Geometry check sheet. Reference: the model listing, model coordinates, mm. A direction names the side the tool comes from. Coordinates: 2 decimals unless noted, no trailing zeros. Loops run counter-clockwise (first coordinate to the right, second up) from the corner with the lowest first, then second, coordinate; pieces in that order, holes last. Notation, with made-up numbers: M 76.5,2 L 125.5,2 A23 ccw 125.5,18 Z; hole C 80.5,38 d4. An arc over 180 degrees is marked long. One line per question, with ' | ' between items. Start each with the question number.
from build123d import *

# Parameters (mm, degrees)
EXTRUDE_354_DEPTH      = 3
CUT_EXTRUDE_1082_REACH = 143.453
SKETCH_3_W             = 15
SKETCH_3_H             = 10
SKETCH_4_R             = 3
SKETCH_4_R_2           = 1.5
EXTRUDE_1381_DEPTH     = 8
SKETCH_5_W             = 83
SKETCH_5_H             = 5
EXTRUDE_1698_DEPTH     = 45
SKETCH_6_W             = 2
SKETCH_6_H             = 5
CUT_EXTRUDE_1867_DEPTH = 83
SKETCH_7_W             = 40
SKETCH_7_H             = 13
TYPE_C_DEPTH           = 3
SKETCH_8_W             = 10
SKETCH_8_H             = 5
CUT_EXTRUDE_3_DEPTH    = 2
SKETCH_9_W             = 11
SKETCH_9_H             = 20
CUT_EXTRUDE_4_DEPTH    = 3
EXTRUDE_START          = -83
EXTRUDE_1_DEPTH        = 83
SKETCH_2_3_R           = 1.5
CUT_EXTRUDE_5_DEPTH    = 10


with BuildPart() as part:
    # 草图1 → Extrude 354 (new body)
    with BuildSketch(Plane(origin=(0, 0, 0), x_dir=(1, 0, 0), z_dir=(0, 1, 0))):
        with BuildLine():
            Line((3, 0), (97, 0))
            ThreePointArc((97, 0), (99.121320344, 0.878679656), (100, 3))
            Line((100, 3), (100, 97))
            ThreePointArc((100, 97), (99.121320344, 99.121320344), (97, 100))
            Line((97, 100), (3, 100))
            ThreePointArc((3, 100), (0.878679656, 99.121320344), (0, 97))
            Line((0, 97), (0, 3))
            ThreePointArc((0, 3), (0.878679656, 0.878679656), (3, 0))
        make_face()
    extrude(amount=EXTRUDE_354_DEPTH)

    # 草图3 → Cut-Extrude 1082 (cut, up to next)
    with BuildSketch(Plane(origin=(0, 3, 0), x_dir=(1, 0, 0), z_dir=(0, 1, 0)), mode=Mode.PRIVATE) as cut_extrude_1082_sk1:
        with Locations((50, 50)):
            Rectangle(SKETCH_3_W, SKETCH_3_H)
    cut_extrude_1082_tool1 = extrude(cut_extrude_1082_sk1.sketch, amount=-CUT_EXTRUDE_1082_REACH, mode=Mode.PRIVATE) & part.part
    add(cut_extrude_1082_tool1.solids().sort_by_distance((50, 3, -50))[0], mode=Mode.SUBTRACT)

    # 草图4 → Extrude 1381 (add)
    with BuildSketch(Plane.XZ):
        with Locations(Location((50, -30, 0), (0, 0, 270))):
            Circle(SKETCH_4_R)
        with Locations(Location((50, -30, 0), (0, 0, 270))):
            Circle(SKETCH_4_R_2, mode=Mode.SUBTRACT)
    extrude(amount=EXTRUDE_1381_DEPTH)

    # 草图5 → Extrude 1698 (add)
    with BuildSketch(Plane.XZ):
        with Locations((50, -97.5)):
            Rectangle(SKETCH_5_W, SKETCH_5_H)
    extrude(amount=EXTRUDE_1698_DEPTH)

    # 草图6 → Cut-Extrude 1867 (cut)
    with BuildSketch(Plane(origin=(91.5, 0, 0), x_dir=(0, 0, -1), z_dir=(1, 0, 0))):
        with Locations((99, -42.5)):
            Rectangle(SKETCH_6_W, SKETCH_6_H)
    extrude(amount=-CUT_EXTRUDE_1867_DEPTH, mode=Mode.SUBTRACT)

    # 草图7 → TYPE-C板口 (cut)
    with BuildSketch(Plane.XY.offset(-95)):
        with Locations((50, -38.5)):
            Rectangle(SKETCH_7_W, SKETCH_7_H)
    extrude(amount=-TYPE_C_DEPTH, mode=Mode.SUBTRACT)

    # 草图8 → 切除-拉伸3 (cut)
    with BuildSketch(Plane.XY.offset(-98)):
        with Locations((50, -37.5)):
            Rectangle(SKETCH_8_W, SKETCH_8_H)
    extrude(amount=-CUT_EXTRUDE_3_DEPTH, mode=Mode.SUBTRACT)

    # 草图9 → 切除-拉伸4 (cut)
    with BuildSketch(Plane.XY.offset(-95)):
        with Locations((86, -17.5)):
            Rectangle(SKETCH_9_W, SKETCH_9_H)
        with Locations((14, -17.5)):
            Rectangle(SKETCH_9_W, SKETCH_9_H)
    extrude(amount=-CUT_EXTRUDE_4_DEPTH, mode=Mode.SUBTRACT)

    # 草图10 → 凸台-拉伸1 (add)
    with BuildSketch(Plane(origin=(91.5, 0, 0), x_dir=(0, 0, -1), z_dir=(1, 0, 0)).offset(EXTRUDE_START)):
        Polygon((95, -7.5), (98, -9.5), (98, -7.5), align=None)
        Polygon((95, -27.5), (98, -25.5), (98, -27.5), align=None)
    extrude(amount=EXTRUDE_1_DEPTH)

    # 放样2: read off the stored shape, not the designer's step
    # 放样2: loft between two sections, ruled curve by curve
    loft_2_from = [
        Edge.make_bspline([(19.446610657, 0, -55.974425515), (31.395461687, 0, -57.081204201), (32.502240373, 0, -45.132353171), (20.553389343, 0, -44.025574485), (8.604538313, 0, -42.918795799), (7.497759627, 0, -54.867646829), (19.446610657, 0, -55.974425515)], [0, 0, 0, 0, 0.5, 0.5, 0.5, 1, 1, 1, 1], 3, [1, 0.333333333, 0.333333333, 1, 0.333333333, 0.333333333, 1]),
    ]
    loft_2_to = [
        Edge.make_bspline([(18.541542898, -10, -52.621622185), (23.784787268, -10, -55.538536389), (26.701701472, -10, -50.295292019), (21.458457102, -10, -47.378377815), (16.215212732, -10, -44.461463611), (13.298298528, -10, -49.704707981), (18.541542898, -10, -52.621622185)], [0, 0, 0, 0, 0.5, 0.5, 0.5, 1, 1, 1, 1], 3, [1, 0.333333333, 0.333333333, 1, 0.333333333, 0.333333333, 1]),
    ]
    loft_2 = Solid(Shell([*[Face.make_surface_from_curves(loft_2_from[k], loft_2_to[k]) for k in range(1)], Face(Wire(loft_2_from)), Face(Wire(loft_2_to))]))
    add(loft_2)

    # 草图2<3> → 切除-拉伸5 (cut)
    with BuildSketch(Plane.XZ.offset(10)):
        with Locations(Location((20, -50, 0), (0, 0, 270))):
            Circle(SKETCH_2_3_R)
    cut_extrude_5 = extrude(amount=-CUT_EXTRUDE_5_DEPTH, mode=Mode.SUBTRACT)

    # 镜向1: 放样2, 切除-拉伸5 across plane
    add(loft_2.mirror(Plane.ZY.offset(-50)))
    add(cut_extrude_5.mirror(Plane.ZY.offset(-50)), mode=Mode.SUBTRACT)


solid = part.part
1. Thickness scan on line 1 (Z direction, x = 80, y = -1.75); line 2 (X direction, y = -7.5, z = -50); line 3 (X direction, y = -6, z = -50). Record the ranges inside material, lowest first.
2. Tool access check on faces 4 (the flat face through (13.9, -26.5, -96.5)), 5 (the flat face through (50, -32, -96)), 6 (the flat face through (91.5, -22, -99)). Record the directions out of +Z, -Z, +X, -X, +Y, -Y that give a thin tool (end or side, any length) a straight path to the whole face; none if there is none.
3. Sectioned sample at C-C (z = -30). Record the cut outline in (x, y).
4. Draft check along Y on faces 1 (the flat face through (19, -45, -96)), 2 (the flat face through (85.9, -26.5, -96.5)), 3 (the flat face through (51, -19, -100)). Enter one of: +Y half, -Y half, draft (parallel to the pull), parting line (faces both ways), or undercut.
5. Sectioned sample at A-A (x = 50). Record the cut outline in (y, z).
6. Depth check by flat-ended pin: pin 1 Ø2.5 at (y, z) = (-33.5, -98.5) entering from +X; pin 2 Ø2 at (x, z) = (50.5, -99) entering from -Y; pin 3 Ø2 at (x, z) = (86, -14) entering from -Y; pin 4 Ø8 at (y, z) = (-15.5, -52.5) entering from -X. Enter the tip coordinate at first touch or a pass-through.
7. Sectioned sample at B-B (x = 12). Record the cut outline in (y, z), and give its area (3 significant figures).
Result:
1) line 1: z = -100 to -95, -55.43 to -51.5, -48.5 to -44.57 | line 2: x = 16.33 to 18.5, 21.5 to 23.67, 76.33 to 78.5, 81.5 to 83.67 | line 3: x = 15.89 to 18.5, 21.5 to 24.11, 75.89 to 78.5, 81.5 to 84.11
2) face 4: +Z, -X | face 5: +Z, -Y | face 6: +Z, -Z, +X, -Y
3) outline: M 0,0 L 47,0 L 47,-8 L 48.5,-8 L 48.5,0 L 51.5,0 L 51.5,-8 L 53,-8 L 53,0 L 100,0 L 100,3 L 0,3 Z
4) face 1: -Y half | face 2: undercut | face 3: draft
5) outline: M -35,-100 L 3,-100 L 3,-55 L 0,-55 L 0,-95 L -32,-95 L -32,-98 L -35,-98 Z; M -8,-33 L 0,-33 L 0,-45 L 3,-45 L 3,0 L 0,0 L 0,-27 L -8,-27 L -8,-28.5 L 0,-28.5 L 0,-31.5 L -8,-31.5 Z
6) pin 1: stops at x = 91.5 | pin 2: stops at y = -35 | pin 3: stops at y = 0 | pin 4: passes through
7) outline: M -45,-98 L -40,-98 L -40,-100 L 3,-100 L 3,0 L 0,0 L 0,-95 L -7.5,-95 L -9.5,-98 L -25.5,-98 L -27.5,-95 L -45,-95 Z | area: 461 mm2
